from build123d import *

# Parameters (mm, degrees)
SKETCH1_R                = 75
BOSS_EXTRUDE1_DEPTH      = 5
SKETCH2_R                = 2.5
CUT_EXTRUDE1_DEPTH       = 5
SKETCH3_R                = 1.4
CUT_EXTRUDE2_DEPTH       = 5
CIRPATTERN1_COUNT        = 4
SKETCH4_W                = 5.5
SKETCH4_H                = 80.5
CUT_EXTRUDE3_DEPTH       = 2.5
SKETCH5_W                = 2.5
SKETCH5_H                = 75
CUT_EXTRUDE4_DEPTH       = 2.5
FILLET1_R                = 0.5
CIRPATTERN2_COUNT        = 2
FILLET1_OF_CIRPATTERN2_R = 0.5


with BuildPart() as part:
    # Sketch1 → Boss-Extrude1 (new body)
    with BuildSketch(Plane(origin=(0, 0, 0), x_dir=(1, 0, 0), z_dir=(0, 1, 0))):
        with Locations(Location((0, 0, 0), (0, 0, 270))):
            Circle(SKETCH1_R)
    extrude(amount=BOSS_EXTRUDE1_DEPTH)

    # Sketch2 → Cut-Extrude1 (cut)
    with BuildSketch(Plane(origin=(0, 5, 0), x_dir=(1, 0, 0), z_dir=(0, 1, 0))):
        with Locations(Location((0, 0, 0), (0, 0, 270))):
            Circle(SKETCH2_R)
    extrude(amount=-CUT_EXTRUDE1_DEPTH, mode=Mode.SUBTRACT)

    # Sketch3 → Cut-Extrude2 (cut)
    with BuildSketch(Plane(origin=(0, 5, 0), x_dir=(1, 0, 0), z_dir=(0, 1, 0))):
        with Locations(Location((0, 12, 0), (0, 0, 270))):
            Circle(SKETCH3_R)
    cut_extrude2 = extrude(amount=-CUT_EXTRUDE2_DEPTH, mode=Mode.SUBTRACT)

    # CirPattern1: Cut-Extrude2 ×4 about axis
    cirpattern1_axis = Axis((0, 0, 0), (0, 1, 0))
    for i in range(1, CIRPATTERN1_COUNT):
        add(cut_extrude2.rotate(cirpattern1_axis, i * 360 / CIRPATTERN1_COUNT), mode=Mode.SUBTRACT)

    # Sketch4 → Cut-Extrude3 (cut)
    with BuildSketch(Plane(origin=(0, 5, 0), x_dir=(1, 0, 0), z_dir=(0, 1, 0))):
        with Locations((-27.5, 0)):
            Rectangle(SKETCH4_W, SKETCH4_H)
    cut_extrude3 = extrude(amount=-CUT_EXTRUDE3_DEPTH, mode=Mode.SUBTRACT)

    # Sketch5 → Cut-Extrude4 (cut)
    with BuildSketch(Plane(origin=(0, 2.5, 0), x_dir=(1, 0, 0), z_dir=(0, 1, 0))):
        with Locations((-27.5, 0)):
            Rectangle(SKETCH5_W, SKETCH5_H)
    cut_extrude4 = extrude(amount=-CUT_EXTRUDE4_DEPTH, mode=Mode.SUBTRACT)

    # Fillet1
    fillet1_edges = [part.edges().sort_by_distance(p)[0] for p in [
        (-24.75, 5, 0),
        (-27.5, 5, -40.25),
        (-30.25, 5, 0),
        (-27.5, 5, 40.25),
    ]]
    fillet(fillet1_edges, radius=FILLET1_R)

    # CirPattern2: Cut-Extrude3, Cut-Extrude4 ×2 about axis
    cirpattern2_axis = Axis((0, 0, 0), (0, 1, 0))
    add([cut_extrude3.rotate(cirpattern2_axis, i * 360 / CIRPATTERN2_COUNT) for i in range(1, CIRPATTERN2_COUNT)], mode=Mode.SUBTRACT)
    add([cut_extrude4.rotate(cirpattern2_axis, i * 360 / CIRPATTERN2_COUNT) for i in range(1, CIRPATTERN2_COUNT)], mode=Mode.SUBTRACT)

    # Fillet1 of CirPattern2
    fillet1_of_cirpattern2_edges = [part.edges().sort_by_distance(p)[0] for p in [
        (24.75, 5, 0),
        (27.5, 5, 40.25),
        (30.25, 5, 0),
        (27.5, 5, -40.25),
    ]]
    fillet(fillet1_of_cirpattern2_edges, radius=FILLET1_OF_CIRPATTERN2_R)


solid = part.part
Input: part model. Units: mm. Frame: model coordinates. A direction names the side the tool comes from. Coordinates: 2 decimals unless noted, no trailing zeros. Write each loop counter-clockwise with the first axis right and the second up, starting at its lowest first coordinate (ties: lowest second). Pieces come first, ordered by that corner, then holes. Notation, with made-up numbers: M 48.25,70.25 L 57.25,70.25 A12 cw 57.25,80.25 Z; hole C -34.75,78 d3. An arc over 180 degrees is marked long. Answer as a JSON object with one key per item and string values. Group by question number.
(1) Ray query, line 1 along X through (y, z) = (2.15, 10); line 2 along X through (y, z) = (1.65, 9.5); line 3 along Z through (x, y) = (-12, 1.15). Return the intervals inside material, ascending. Write a range as [from, to].
(2) Set-up query: faces 4 (the face through (-2.44, 2.54, -0.54)), 5 (the face through (29, 2.5, 1)). Return all of +Z, -Z, +X, -X, +Y, -Y with unobstructed straight access to the full face (end or side cutting, diameter ignored); none if empty.
(3) Contact query for flat-ended pins moving along their axis: P1, Ø3, axis at x = -43, z = 15, coming from the -Y side; P2, Ø2, axis at x = -28.5, y = 4.5, coming from the -Z side; P3, Ø1.2, axis at y = 1.5, z = 4.5, coming from the +X side; P4, Ø2.5, axis at x = 0, z = -12, coming from the -Y side. Output: stop coordinate, or through.
(4) Section C-C on z = 45. Output: boundary loops of the cut face in (x, y), plus the area to 3 significant figures.
(5) Section B-B on z = 28. Output: boundary loops of the cut face in (x, y), plus the area to 3 significant figures.
(6) Section A-A on y = 1.65. Output: boundary loops of the cut face in (x, z).
(7) Section D-D on x = -17.5. Output: boundary loops of the cut face in (y, z).
(8) Mould query, pull axis X, two halves, no side actions, for faces 1 (the face through (-29, 2.5, -1)), 2 (the face through (-16, 0, -1)), 3 (the face through (-45.636, 2.465, -59.517)). Classes: pulls with the +X half, pulls with the -X half, needs draft (parallel to the pull), parting line crosses it, or undercut.
Result set:
{
 "1": {"line 1": "x = [-74.33, -28.75], [-26.25, 26.25], [28.75, 74.33]", "line 2": "x = [-74.4, -28.75], [-26.25, 26.25], [28.75, 74.4]", "line 3": "z = [-74.03, -1.4], [1.4, 74.03]"},
 "2": {"face 4": "+Y, -Y", "face 5": "+Y"},
 "3": {"P1": "stops at y = 0", "P2": "stops at z = -69.78", "P3": "stops at x = 74.9", "P4": "passes through"},
 "4": {"outline": "M -60,0 L 60,0 L 60,5 L -60,5 Z", "area": "600 mm2"},
 "5": {"outline": "M -69.58,0 L -28.75,0 L -28.75,2.5 L -30.25,2.5 L -30.25,4.5 A0.5 ccw -30.75,5 L -69.58,5 Z; M -26.25,0 L 26.25,0 L 26.25,2.5 L 24.75,2.5 L 24.75,4.5 A0.5 ccw 24.25,5 L -24.25,5 A0.5 ccw -24.75,4.5 L -24.75,2.5 L -26.25,2.5 Z; M 28.75,0 L 69.58,0 L 69.58,5 L 30.75,5 A0.5 ccw 30.25,4.5 L 30.25,2.5 L 28.75,2.5 Z", "area": "656 mm2"},
 "6": {"outline": "C 0,0 d150; hole M -28.75,-37.5 L -26.25,-37.5 L -26.25,37.5 L -28.75,37.5 Z; hole C -12,0 d2.8; hole C 0,0 d5; hole C 0,-12 d2.8; hole C 0,12 d2.8; hole C 12,0 d2.8; hole M 26.25,-37.5 L 28.75,-37.5 L 28.75,37.5 L 26.25,37.5 Z"},
 "7": {"outline": "M 0,-72.93 L 5,-72.93 L 5,72.93 L 0,72.93 Z"},
 "8": {"face 1": "undercut", "face 2": "needs draft", "face 3": "parting line crosses it"}
}
